Build history of the part. All positions in model axes, mm. Face numbers are marked on the shaded views. Give positions to 0.01 mm unless a question says otherwise; leave off trailing zeros. Loops run counter-clockwise (first coordinate to the right, second up) from the corner with the lowest first, then second, coordinate; pieces in that order, holes last.
1) Wall check: line 1 (Y direction, x = -12.7, z = -1.2) (3 decimals); line 2 (Z direction, x = -23.25, y = 347). Give the ranges that are in metal, low to high.
2) Flat gauge pins, fed straight in: P1, Ø11.5, axis at x = -13.97, y = 151.892, coming from the -Z side; P2, Ø4, axis at x = -12.7, y = 622.3, coming from the +Z side. Where does each tip first touch, or does it go through?
3) Two-plate mould, pull along Z, no slides. Class the marked faces 1 and 2: +Z half, -Z half, draft (parallel to the pull), parting line (faces both ways), or undercut.
4) Band-saw the part on B-B on y = 12.7. List the corners of the cut face in (x, z), then the cut area to 3 significant figures.
5) Band-saw the part on C-C on y = 506. List the corners of the cut face in (x, z).
6) Band-saw the part on A-A on z = -12. List the corners of the cut face in (x, y), then the cut area to 3 significant figures.
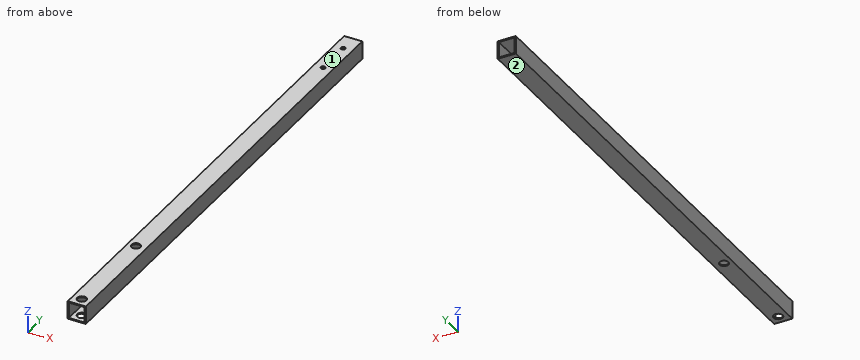
Autodesk Inventor part; units mm, degrees
ref_plane "YZ Plane" through (0, 0, 0) normal (1, 0, 0) x (0, 1, 0)
ref_plane "XZ Plane" through (0, 0, 0) normal (0, 1, 0) x (-1, 0, 0)
ref_plane "XY Plane" through (0, 0, 0) normal (0, 0, 1) x (1, 0, 0)
sketch "Sketch1" plane through (0, 0, 0) normal (0, 1, 0) x (-1, 0, 0)
  line L0 (0, 0) -> (25.4, 0)
  line L1 (25.4, 0) -> (25.4, -25.4)
  line L2 (25.4, -25.4) -> (0, -25.4)
  line L3 (0, -25.4) -> (0, 0)
  line L4 (23.8125, -23.8125) -> (23.8125, -1.5875)
  line L5 (23.8125, -1.5875) -> (1.5875, -1.5875)
  line L6 (1.5875, -1.5875) -> (1.5875, -23.8125)
  line L7 (1.5875, -23.8125) -> (23.8125, -23.8125)
  dimension "d0" = 25.4
  dimension "d1" = 25.4
  dimension "d2" = 1.5875
extrude "Extrusion1" add sketch "Sketch1" along normal blind 698.5
sketch "Sketch2" plane through (-25.4, 0, 0) normal (0, 0, 1) x (1, 0, 0)
  circle A0 centre (12.7, 12.7) radius 6.35
  line L0 (25.4, 0) -> (0, 0)
  dimension "d5" = 12.7
  dimension "d6" = 12.7
extrude "Extrusion2" cut sketch "Sketch2" against normal blind 25.4
sketch "Sketch7" plane through (0, 0, -25.4) normal (0, 0, -1) x (-1, 0, 0)
  circle A0 centre (13.97, 151.892) radius 6.35
  line L0 (25.4, 0) -> (0, 0)
  line L1 (25.4, 0) -> (25.4, 698.5)
  dimension "d26" = 12.7
  dimension "d27" = 151.892
  dimension "d31" = 11.43
extrude "Extrusion7" cut sketch "Sketch7" against normal blind 25.4
sketch "Sketch11" plane through (0, 0, -25.4) normal (0, 0, -1) x (-1, 0, 0)
  line L0 (0, 698.5) -> (25.4, 698.5)
  line L1 (0, 0) -> (0, 698.5)
  line L2 (0, 723.9) -> (0, 669.7136)
  arc A0 (0, 669.7136) -> (-29.6572, 670.9249) centre (-16.2109, 636.4744) ccw
  line L3 (-29.6572, 670.9249) -> (-33.1564, 670.9249)
  line L4 (-29.6572, 670.9249) -> (-33.1564, 670.9249)
  arc A1 (0, 669.7136) -> (-29.6572, 670.9249) centre (-16.2109, 636.4744) ccw
  arc A2 (0, 723.9) -> (-33.1564, 670.9249) centre (3.7035, 684.7184) ccw
  point P0 (25.4, 698.5)
extrude "Extrusion11" cut sketch "Sketch11" against normal blind 25.4
sketch "Sketch12" plane through (-25.4, 0, 0) normal (0, 0, 1) x (1, 0, 0)
  line L0 (25.4, 698.5) -> (0, 698.5)
  circle A0 centre (12.7, 673.1) radius 3.175
  circle A1 centre (12.7, 622.3) radius 3.175
  point P0 (25.4, 0)
  dimension "d46" = 6.35
  dimension "d47" = 25.4
  dimension "d48" = 6.35
  dimension "d50" = 76.2
extrude "Extrusion12" cut sketch "Sketch12" against normal blind 1.5875
properties part number "AP 3"
Findings below:
1. line 1: y = 0 to 6.35, 19.05 to 145.67, 158.114 to 619.125, 625.475 to 669.925, 676.275 to 698.5
1. line 2: z = -25.4 to -23.81, -1.59 to 0
2. P1: passes through
2. P2: stops at z = -23.81
3. face 1: +Z half
3. face 2: -Z half
4. outline: (-25.4, -25.4) - (-19.05, -25.4) - (-19.05, -23.81) - (-23.81, -23.81) - (-23.81, -1.59) - (-19.05, -1.59) - (-19.05, 0) - (-25.4, 0) - close; (-6.35, -25.4) - (0, -25.4) - (0, 0) - (-6.35, 0) - (-6.35, -1.59) - (-1.59, -1.59) - (-1.59, -23.81) - (-6.35, -23.81) - close
4. area: 111 mm2
5. outline: (-25.4, -25.4) - (0, -25.4) - (0, 0) - (-25.4, 0) - close; hole (-23.81, -23.81) - (-1.59, -23.81) - (-1.59, -1.59) - (-23.81, -1.59) - close
6. outline: (-25.4, 0) - (-23.81, 0) - (-23.81, 698.5) - (-25.4, 698.5) - close; (-1.59, 0) - (0, 0) - (0, 698.5) - (-1.59, 698.5) - close
6. area: 2,220 mm2
